```python
from build123d import *

# Parameters (mm, degrees)
BOSS_EXTRUDE1_DEPTH     = 6.35
SKETCH3_R               = 1.5875
CUT_EXTRUDE1_DEPTH      = 12.696129591
CUT_EXTRUDE1_DEPTH_BACK = 11.834286606
SKETCH4_W               = 3.175
SKETCH4_H               = 7.9375
BOSS_EXTRUDE3_DEPTH     = 6.35
SKETCH5_R               = 3.81
CUT_EXTRUDE2_DEPTH      = 7.540625
SKETCH6_R               = 1.5875
CUT_EXTRUDE3_DEPTH      = 15.2875
SKETCH7_W               = 3.571875
SKETCH7_H               = 3.175
CUT_EXTRUDE4_DEPTH      = 13.7
BOSS_EXTRUDE4_DEPTH     = 3.175
CUT_EXTRUDE5_DEPTH      = 13.039014125
CUT_EXTRUDE5_DEPTH_BACK = 4.175


with BuildPart() as part:
    # Sketch2 → Boss-Extrude1 (new body, symmetric)
    with BuildSketch(Plane.XY):
        with BuildLine():
            Line((-14.2875, -1.570977871), (-18.32092114, -5.604399011))
            ThreePointArc((-18.32092114, -5.604399011), (-18.32092114, -7.849463042), (-16.07585711, -7.849463042))
            Line((-16.07585711, -7.849463042), (-11.1125, -2.886105932))
            Line((-11.1125, -2.886105932), (-11.1125, 1.5875))
            Line((-11.1125, 1.5875), (0, 1.5875))
            Line((0, 1.5875), (0, 4.7625))
            Line((0, 4.7625), (-14.2875, 4.7625))
            Line((-14.2875, 4.7625), (-14.2875, -1.570977871))
        make_face()
    extrude(amount=BOSS_EXTRUDE1_DEPTH, both=True)

    # Sketch3 → Cut-Extrude1 (cut, two sides)
    with BuildSketch(Plane(origin=(-4.113197034, 4.113197034, 0), x_dir=(0, 0, -1), z_dir=(0.707106781, -0.707106781, 0))) as cut_extrude1_sk:
        with Locations((0, -13.742756121)):
            Circle(SKETCH3_R)
    extrude(amount=CUT_EXTRUDE1_DEPTH, mode=Mode.SUBTRACT)
    extrude(cut_extrude1_sk.sketch, amount=-CUT_EXTRUDE1_DEPTH_BACK, mode=Mode.SUBTRACT)

    # Sketch4 → Boss-Extrude3 (add, symmetric)
    with BuildSketch(Plane.XY):
        with Locations((-5.159375, 5.55625)):
            Rectangle(SKETCH4_W, SKETCH4_H)
    extrude(amount=BOSS_EXTRUDE3_DEPTH, both=True)

    # Sketch5 → Cut-Extrude2 (cut)
    with BuildSketch(Plane.ZY.offset(14.2875)):
        with Locations((0, 4.7625)):
            Circle(SKETCH5_R)
    extrude(amount=-CUT_EXTRUDE2_DEPTH, mode=Mode.SUBTRACT)

    # Sketch6 → Cut-Extrude3 (cut, through all)
    with BuildSketch(Plane.ZY.offset(14.2875)):
        with Locations((0, 4.7625)):
            Circle(SKETCH6_R)
    extrude(amount=-CUT_EXTRUDE3_DEPTH, mode=Mode.SUBTRACT)

    # Sketch7 → Cut-Extrude4 (cut, through all)
    with BuildSketch(Plane.XY.offset(6.35)):
        with Locations((-1.7859375, 3.175)):
            Rectangle(SKETCH7_W, SKETCH7_H)
    extrude(amount=-CUT_EXTRUDE4_DEPTH, mode=Mode.SUBTRACT)

    # Sketch8 → Boss-Extrude4 (add)
    with BuildSketch(Plane(origin=(-3.571875, 0, 0), x_dir=(0, 0, -1), z_dir=(1, 0, 0))):
        with BuildLine():
            ThreePointArc((6.35, 12.7), (0, 19.05), (-6.35, 12.7))
            ThreePointArc((-6.35, 12.7), (-6.133628997, 11.056499064), (-5.499261314, 9.525))
            Line((-5.499261314, 9.525), (5.499261314, 9.525))
            ThreePointArc((5.499261314, 9.525), (6.133628997, 11.056499064), (6.35, 12.7))
        make_face()
        with BuildLine():
            Line((5.499261314, 9.525), (-5.499261314, 9.525))
            ThreePointArc((-5.499261314, 9.525), (0, 6.35), (5.499261314, 9.525))
        make_face()
        with BuildLine():
            Line((-6.35, 12.7), (-6.35, 9.525))
            Line((-6.35, 9.525), (-5.499261314, 9.525))
            ThreePointArc((-5.499261314, 9.525), (-6.133628997, 11.056499064), (-6.35, 12.7))
        make_face()
        with BuildLine():
            Line((6.35, 9.525), (6.35, 12.7))
            ThreePointArc((6.35, 12.7), (6.133628997, 11.056499064), (5.499261314, 9.525))
            Line((5.499261314, 9.525), (6.35, 9.525))
        make_face()
    extrude(amount=-BOSS_EXTRUDE4_DEPTH)

    # Sketch9 → Cut-Extrude5 (cut, two sides)
    with BuildSketch(Plane.ZY.offset(6.746875)) as cut_extrude5_sk:
        with BuildLine():
            ThreePointArc((-2.404382567, 13.757225005), (0, 11.912277372), (2.404382567, 13.757225005))
            Line((2.404382567, 13.757225005), (0, 14.401477372))
            Line((0, 14.401477372), (-2.404382567, 13.757225005))
        make_face()
        with BuildLine():
            Line((0, 14.401477372), (2.404382567, 13.757225005))
            ThreePointArc((2.404382567, 13.757225005), (2.467904549, 14.076571574), (2.4892, 14.401477372))
            ThreePointArc((2.4892, 14.401477372), (2.467904549, 14.72638317), (2.404382567, 15.045729739))
            Line((2.404382567, 15.045729739), (0, 14.401477372))
        make_face()
        with BuildLine():
            Line((-2.404382567, 13.757225005), (0, 14.401477372))
            Line((0, 14.401477372), (-2.404382567, 15.045729739))
            ThreePointArc((-2.404382567, 15.045729739), (-2.4892, 14.401477372), (-2.404382567, 13.757225005))
        make_face()
        with BuildLine():
            Line((-2.404382567, 15.045729739), (0, 14.401477372))
            Line((0, 14.401477372), (2.404382567, 15.045729739))
            ThreePointArc((2.404382567, 15.045729739), (0, 16.890677372), (-2.404382567, 15.045729739))
        make_face()
    extrude(amount=CUT_EXTRUDE5_DEPTH, mode=Mode.SUBTRACT)
    extrude(cut_extrude5_sk.sketch, amount=-CUT_EXTRUDE5_DEPTH_BACK, mode=Mode.SUBTRACT)


solid = part.part
```
For this review, take the finished solid that the model builds, in its own axes (mm). A direction names the side the tool comes from. Coordinates: 2 decimals unless noted, no trailing zeros. Write each loop counter-clockwise with the first axis right and the second up, starting at its lowest first coordinate (ties: lowest second). Pieces come first, ordered by that corner, then holes. Notation, with made-up numbers: (80.25, 40) - (133.25, 40) arc R7 ccw to (133.25, 46) - close; hole circle Ø7 at (62, 47). An arc over 180 degrees is marked (long way). Answer in a Markdown table with one row per item. Add a question column.
Q1. Tool access review of faces 4 (the cylindrical face through (-11.408, 0.953, -0.084)), 5 (the flat face through (-14.288, 0, 0)), 6 (the flat face through (-3.572, 10, 0)), 7 (the flat face through (-6.56, 1.588, 0.09)): name each direction out of +Z, -Z, +X, -X, +Y, -Y from which nothing blocks a thin tool from reaching the whole face with its end or side.
Q2. We need section D-D, the plane y = 13.25. State the section outline as (x, z) points.
Q3. For P1, Ø2, axis at y = 12, z = 0, coming from the -X side; P2, Ø2, axis at x = -6.5, y = 13.5, coming from the -Z side; P3, Ø4, axis at x = -8.5, z = -1.5, coming from the -Y side; P4, Ø1.5, axis at x = -15.5, y = 1, coming from the -Z side, all flat-tipped, find the tip position at first contact; note any pin that passes through.
Q4. We need section B-B, the plane z = 0. Count the separate pieces of the cut face and the enclosed holes in it, and give its area (3 significant figures).
Q5. For probe 1 along X at (y, z) = (8.5, -3.75); probe 2 along Z at (x, y) = (-14.25, 4); probe 3 along X at (y, z) = (-0.25, 0.25), list the stretches that pass through material, from the lowest coordinate up.
Q6. We need section A-A, the plane x = -8.25. State the section outline as (y, z) points.
Q7. Draft analysis for pull direction Y (two halves, no side actions). For faces 1 (the cylindrical face through (-18.35, -7.82, 0.09)), 2 (the cylindrical face through (-13.825, -3.385, 0.207)), 3 (the flat face through (-11.112, -1, 0)), state which applies: +Y half, -Y half, draft (parallel to the pull), parting line (faces both ways), or undercut.
Answer list:
| question | item | result |
|---|---|---|
| 1 | face 4 | -X, +Y |
| 1 | face 5 | +Z, -Z, -X, +Y |
| 1 | face 6 | +Z, -Z, +X, +Y, -Y |
| 1 | face 7 | +Z, -Z, +X, -Y |
| 2 | outline | (-6.75, -6.33) - (-3.57, -6.33) - (-3.57, -2.21) - (-6.75, -2.21) - close; (-6.75, 2.21) - (-3.57, 2.21) - (-3.57, 6.33) - (-6.75, 6.33) - close |
| 3 | P1 | stops at x = -6.75 |
| 3 | P2 | stops at z = -6.35 |
| 3 | P3 | stops at y = 1.59 |
| 3 | P4 | passes through |
| 4 | separate pieces | 5 |
| 4 | enclosed holes | 0 |
| 4 | area | 53.7 mm2 |
| 5 | probe 1 | x = -6.75 to -3.57 |
| 5 | probe 2 | z = -6.35 to -3.73, 3.73 to 6.35 |
| 5 | probe 3 | x = -14.29 to -11.11 |
| 6 | outline | (1.59, -6.35) - (4.76, -6.35) - (4.76, -3.81) arc R3.81 cw to (1.59, -2.11) - close; (1.59, 2.11) arc R3.81 cw to (4.76, 3.81) - (4.76, 6.35) - (1.59, 6.35) - close |
| 7 | face 1 | parting line |
| 7 | face 2 | undercut |
| 7 | face 3 | draft |
